```python
from build123d import *

# Parameters (mm, degrees)
F0_W      = 125
F0_H      = 100
F0_W_2    = 66.56
F0_H_2    = 57
F1_DEPTH  = 7.5
F2_W      = 174.649224
F2_H      = 78.5
F3_DEPTH  = 4.75
F4_W      = 2.74
F4_H      = 78.5
F5_DEPTH  = 1.5
F6_W      = 7.8
F6_H      = 78.5
F7_DEPTH  = 4.75
F8_W      = 7.8
F8_H      = 100
F9_DEPTH  = 25
F10_R     = 1.5
F11_DEPTH = 25
F12_R     = 1.5
F13_DEPTH = 25


with BuildPart() as f1:
    # F0 (on Front) → F1 (new body)
    with BuildSketch(Plane.XZ):
        Rectangle(F0_W, F0_H)
        Rectangle(F0_W_2, F0_H_2, mode=Mode.SUBTRACT)
    extrude(amount=F1_DEPTH)

    # F2 (on face) → F3 (cut)
    with BuildSketch(Plane.XZ.offset(7.5)):
        Rectangle(F2_W, F2_H)
    extrude(amount=-F3_DEPTH, mode=Mode.SUBTRACT)

    # F4 (on face) → F5 (cut)
    with BuildSketch(Plane.XZ.offset(2.75)):
        with Locations((44.69, 0)):
            Rectangle(F4_W, F4_H)
    extrude(amount=-F5_DEPTH, mode=Mode.SUBTRACT)

    # F6 (on face) → F7 (join)
    with BuildSketch(Plane.XZ.offset(2.75)):
        with Locations((-58.6, 0)):
            Rectangle(F6_W, F6_H)
    extrude(amount=F7_DEPTH)

    # F8 (on face) → F9 (cut)
    with BuildSketch(Plane.XZ.offset(7.5)):
        with Locations((-58.6, 0)):
            Rectangle(F8_W, F8_H)
    extrude(amount=-F9_DEPTH, mode=Mode.SUBTRACT)

    # F10 (on face) → F11 (cut)
    with BuildSketch(Plane.XZ.offset(7.5)):
        with Locations((0, 44.625)):
            Circle(F10_R)
        with Locations((-35, 44.625)):
            Circle(F10_R)
        with Locations((35, 44.625)):
            Circle(F10_R)
    extrude(amount=-F11_DEPTH, mode=Mode.SUBTRACT)

    # F12 (on face) → F13 (cut)
    with BuildSketch(Plane.XZ.offset(7.5)):
        with Locations((0, -44.625)):
            Circle(F12_R)
        with Locations((35, -44.625)):
            Circle(F12_R)
        with Locations((-35, -44.625)):
            Circle(F12_R)
    extrude(amount=-F13_DEPTH, mode=Mode.SUBTRACT)


solid = f1.part
```
Input: part model. Units: mm. Frame: model coordinates. A direction names the side the tool comes from. Coordinates: 2 decimals unless noted, no trailing zeros. Loops run counter-clockwise (first coordinate to the right, second up) from the corner with the lowest first, then second, coordinate; pieces in that order, holes last. Notation, with made-up numbers: M 34,77.25 L 56,77.25 A21 ccw 56,92.25 Z; hole C 55,63 d4. An arc over 180 degrees is marked long. One line per item, written item: value.
(1) Pin query (flat end, axial travel): pin 1 (13 mm diameter, centred on x = 56, z = 16, fed in from -Y). Return the tip coordinate at first contact, or that it passes through.
Filled in:
pin 1: y = -2.75
(2) Section B-B (y = -6.25). Output: boundary loops of the cut face in (x, z) (3 decimals), and give its area (3 significant figures).
Filled in:
outline: M -54.7,-50 L 62.5,-50 L 62.5,-39.25 L -54.7,-39.25 Z; M -54.7,39.25 L 62.5,39.25 L 62.5,50 L -54.7,50 Z; hole C -35,-44.625 d3; hole C -35,44.625 d3; hole C 0,-44.625 d3; hole C 0,44.625 d3; hole C 35,-44.625 d3; hole C 35,44.625 d3
area: 2,480 mm^2
(3) Line query: line 1 along Z through (x, y) = (-35, -4.5) (3 decimals); line 2 along X through (y, z) = (-2, -5.5); line 3 along X through (y, z) = (-6, 44.5). Output: solid intervals per line, ascending. Write a range as from..to.
Filled in:
line 1: -50..-46.125, -43.125..-39.25, 39.25..43.125, 46.125..50
line 2: -54.7..-33.28, 33.28..43.32, 46.06..62.5
line 3: -54.7..-36.49, -33.51..-1.49, 1.49..33.51, 36.49..62.5
(4) Pull-direction query (X, two-part tool) for faces 1 (the flat face through (33.28, -1, 0)), 2 (the flat face through (-39, -2.75, 1)), 3 (the flat face through (62.5, -2, -1)), 4 (the cylindrical face through (34.67, -3.8, 43.16)); classes: +X half, -X half, draft (parallel to the pull), parting line (faces both ways), or undercut.
Filled in:
face 1: undercut
face 2: draft
face 3: +X half
face 4: undercut
(5) Reachability of faces 5 (the flat face through (3, -4, 50)), 6 (the flat face through (-33.28, -1, 0)), 7 (the flat face through (54, -2.75, 1)) from +Z, -Z, +X, -X, +Y, -Y: full face, straight path, thin tool, end or side. Return the list, or none.
Filled in:
face 5: +Z, +X, -X, +Y, -Y
face 6: +Y, -Y
face 7: +X, -X, -Y
(6) Section D-D (x = 7). Output: boundary loops of the cut face in (y, z).
Filled in:
outline: M -7.5,-50 L 0,-50 L 0,-28.5 L -2.75,-28.5 L -2.75,-39.25 L -7.5,-39.25 Z; M -7.5,39.25 L -2.75,39.25 L -2.75,28.5 L 0,28.5 L 0,50 L -7.5,50 Z
(7) Section C-C (x = 35). Output: boundary loops of the cut face in (y, z) (3 decimals).
Filled in:
outline: M -7.5,-50 L 0,-50 L 0,-46.125 L -7.5,-46.125 Z; M -7.5,-43.125 L 0,-43.125 L 0,43.125 L -7.5,43.125 L -7.5,39.25 L -2.75,39.25 L -2.75,-39.25 L -7.5,-39.25 Z; M -7.5,46.125 L 0,46.125 L 0,50 L -7.5,50 Z
(8) Section A-A (z = 8). Output: boundary loops of the cut face in (x, y), and give its area (3 significant figures).
Filled in:
outline: M -54.7,-2.75 L -33.28,-2.75 L -33.28,0 L -54.7,0 Z; M 33.28,-2.75 L 43.32,-2.75 L 43.32,-1.25 L 46.06,-1.25 L 46.06,-2.75 L 62.5,-2.75 L 62.5,0 L 33.28,0 Z
area: 135 mm^2
